Can you work these out from the model? Positions are in its coordinate system, mm. A direction names the side the tool comes from. Round coordinates to 2 decimals unless told otherwise and drop trailing zeros. Write each loop counter-clockwise with the first axis right and the second up, starting at its lowest first coordinate (ties: lowest second). Pieces come first, ordered by that corner, then holes.
Q1. If we section it at D-D (z = 17.5): Please give me the cut outline in (x, y), plus the area to 3 significant figures.
Q2. Please list where these lines run through material, in increasing order: line 1 along X through (y, z) = (4, 52.5); line 2 along Z through (x, y) = (23.5, 3); line 3 along X through (y, z) = (11.75, 8).
Q3. For faces 1 (the flat face through (35.42, 13, 13)), 2 (the flat face through (37.513, 13, 13)), 3 (the flat face through (85, 4, 28)), which set-ups out of +Z, -Z, +X, -X, +Y, -Y let a thin tool reach every point of the face, with its end or its side?
Q4. If we section it at A-A (x = 23.5): Please give me the cut outline in (y, z), plus the area to 3 significant figures.
Q5. If we section it at C-C (y = 13): Please give me the cut outline in (x, z), plus the area to 3 significant figures.
Q6. I'm going to push flat-ended pins straight in: pin 1 Ø17 at (x, z) = (44, 41) entering from +Y; pin 2 Ø0.6 at (x, y) = (36, 13.5) entering from -Z; pin 3 Ø2.5 at (y, z) = (12.5, 29.5) entering from +X; pin 4 Ø2 at (x, z) = (23.5, 52.5) entering from +Y. Where does each tip first touch, or does it pass through?
Q7. If we section it at B-B (z = 3.5): Please give me the cut outline in (x, y), plus the area to 3 significant figures.
Q8. We'd pull the mould along Z, two halves only. Please class faces 4 (the flat face through (36, 13, 23.469)), 5 (the cylindrical face through (82.12, 4.44, 53.7)), 6 (the flat face through (36, 13, 1.469)), 7 (the flat face through (0, 9, 28)): +Z half, -Z half, draft (parallel to the pull), parting line (faces both ways), or undercut.
from build123d import *

# Parameters (mm, degrees)
SKETCH1_W             = 20
SKETCH1_H             = 56
BOSS_EXTRUDE1_DEPTH   = 18
SKETCH1_W_2           = 2.09336208
SKETCH1_H_2           = 22
BOSS_EXTRUDE1_2_DEPTH = 18
SKETCH1_3_W           = 65
SKETCH1_3_H           = 56
SKETCH1_3_R           = 1.35
SKETCH1_3_W_2         = 2.09336208
SKETCH1_3_H_2         = 22
BOSS_EXTRUDE2_DEPTH   = 9


with BuildPart() as part:
    # Sketch1 → Boss-Extrude1 (new body)
    with BuildSketch(Plane(origin=(0, 0, 0), x_dir=(1, 0, 0), z_dir=(0, 1, 0))):
        with Locations((10, -28)):
            Rectangle(SKETCH1_W, SKETCH1_H)
    extrude(amount=BOSS_EXTRUDE1_DEPTH)



with BuildPart() as body_2:
    # Sketch1 → Boss-Extrude1 2 (new body)
    with BuildSketch(Plane(origin=(0, 0, 0), x_dir=(1, 0, 0), z_dir=(0, 1, 0))):
        with Locations((36.46668104, -12.469488465)):
            Rectangle(SKETCH1_W_2, SKETCH1_H_2)
    extrude(amount=BOSS_EXTRUDE1_2_DEPTH)


with BuildPart() as part_1:
    add(part.part)

    add(body_2.part)  # Boss-Extrude2 merges body 2
    # Sketch1<3> → Boss-Extrude2 (add)
    with BuildSketch(Plane(origin=(0, 0, 0), x_dir=(1, 0, 0), z_dir=(0, 1, 0))):
        with Locations((52.5, -28)):
            Rectangle(SKETCH1_3_W, SKETCH1_3_H)
        with Locations((23.5, -52.5)):
            Circle(SKETCH1_3_R, mode=Mode.SUBTRACT)
        with Locations((81.5, -52.5)):
            Circle(SKETCH1_3_R, mode=Mode.SUBTRACT)
        with Locations((36.46668104, -12.469488465)):
            Rectangle(SKETCH1_3_W_2, SKETCH1_3_H_2, mode=Mode.SUBTRACT)
        with Locations((23.5, -3.5)):
            Circle(SKETCH1_3_R, mode=Mode.SUBTRACT)
        with Locations((81.5, -3.5)):
            Circle(SKETCH1_3_R, mode=Mode.SUBTRACT)
    extrude(amount=BOSS_EXTRUDE2_DEPTH)


solid = part_1.part
A:
1. outline: (0, 0) - (85, 0) - (85, 9) - (37.51, 9) - (37.51, 18) - (35.42, 18) - (35.42, 9) - (20, 9) - (20, 18) - (0, 18) - close
1. area: 964 mm2
2. line 1: x = 0 to 22.15, 24.85 to 80.15, 82.85 to 85
2. line 2: z = 0 to 2.15, 4.85 to 51.15, 53.85 to 56
2. line 3: x = 0 to 20, 35.42 to 37.51
3. face 1: +Z, -Z, +Y
3. face 2: +Z, -Z, +X, +Y
3. face 3: +Z, -Z, +X, +Y, -Y
4. outline: (0, 0) - (9, 0) - (9, 2.15) - (0, 2.15) - close; (0, 4.85) - (9, 4.85) - (9, 51.15) - (0, 51.15) - close; (0, 53.85) - (9, 53.85) - (9, 56) - (0, 56) - close
4. area: 455 mm2
5. outline: (0, 0) - (20, 0) - (20, 56) - (0, 56) - close; (35.42, 1.47) - (37.51, 1.47) - (37.51, 23.47) - (35.42, 23.47) - close
5. area: 1,170 mm2
6. pin 1: stops at y = 9
6. pin 2: stops at z = 1.47
6. pin 3: stops at x = 20
6. pin 4: passes through
7. outline: (0, 0) - (22.15, 0) - (22.15, 9) - (20, 9) - (20, 18) - (0, 18) - close; (24.85, 0) - (80.15, 0) - (80.15, 9) - (37.51, 9) - (37.51, 18) - (35.42, 18) - (35.42, 9) - (24.85, 9) - close; (82.85, 0) - (85, 0) - (85, 9) - (82.85, 9) - close
7. area: 915 mm2
8. face 4: +Z half
8. face 5: undercut
8. face 6: -Z half
8. face 7: draft
